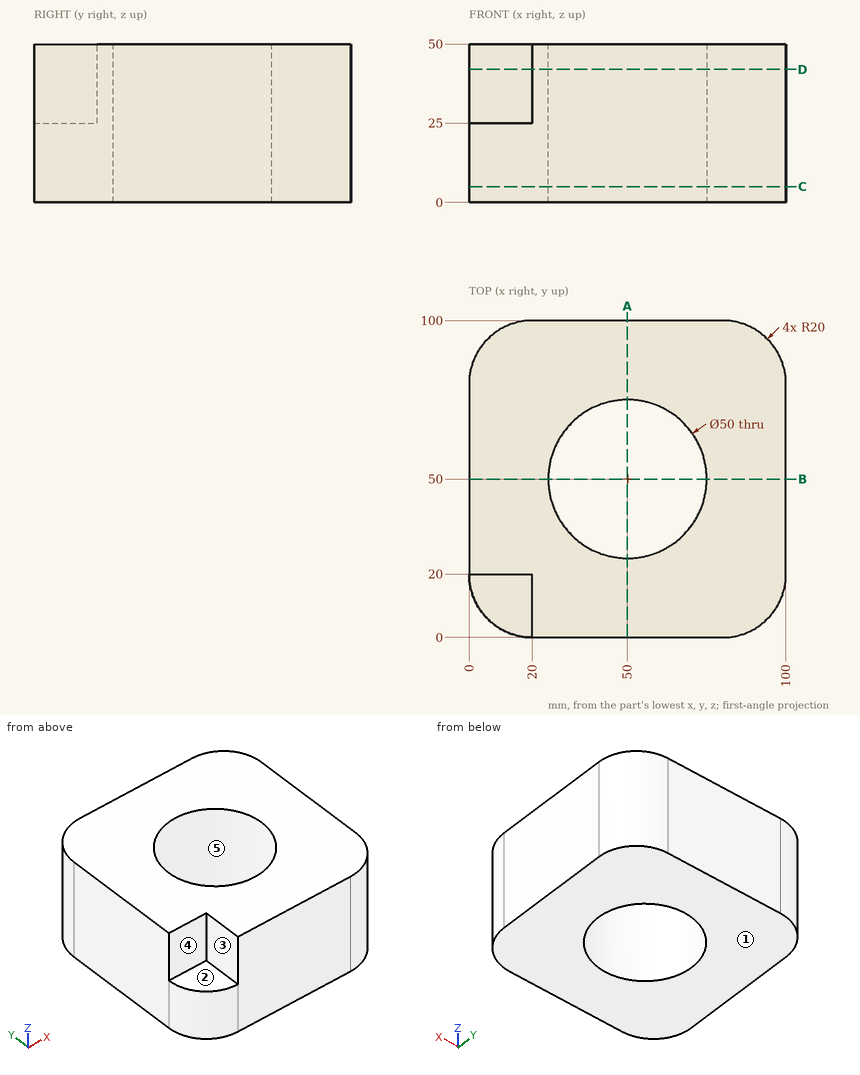
Verification items for this drawing (mm, ordinates from the low corner). A direction names the side the tool comes from. Give positions to 0.01 mm unless a question says otherwise; leave off trailing zeros. Loops run counter-clockwise (first coordinate to the right, second up) from the corner with the lowest first, then second, coordinate; pieces in that order, holes last. Notation, with made-up numbers: M 16.25,86 L 56.25,86 A16 cw 56.25,102 Z; hole C 84.25,-35.5 d3. An arc over 180 degrees is marked long. Answer as a JSON object with one key per item and string values. Group by question number.
Q1. Go/stop test with flat-tipped pins: P1, Ø6, axis at x = 7.5, y = 6.5, coming from the +Z side; P2, Ø12, axis at y = 11, z = 36, coming from the +X side; P3, Ø6, axis at x = 11.5, z = 36, coming from the -Y side. Record where each tip stops, or that it passes through.
Q2. Release check for a two-part mould opening along X. For the marked faces 3, 4 and 5 record: released by +X, released by -X, zero draft, split by the parting line, or undercut.
Q3. Access from +Z, -Z, +X, -X, +Y, -Y to the whole of each face (thin tool, end or side, straight path). Record for the marked faces 1 and 2.
Q4. Cross-section at A-A on x = 50. Record the cut outline in (y, z).
Q5. Material ranges on line 1 along Y through (x, z) = (50, 35.5); line 2 along X through (y, z) = (40.5, 35.5); line 3 along X through (y, z) = (65, 19), recorded low to high. Write a range as [from, to].
Q6. Cross-section at C-C on z = 5. Record the cut outline in (x, y), then the cut area to 3 significant figures.
Q7. Cross-section at D-D on z = 42. Record the cut outline in (x, y), then the cut area to 3 significant figures.
Evaluation:
{
 "1": {"P1": "stops at z = 25", "P2": "stops at x = 99.77", "P3": "stops at y = 20"},
 "2": {"face 3": "released by -X", "face 4": "zero draft", "face 5": "undercut"},
 "3": {"face 1": "-Z, +X, -X, +Y, -Y", "face 2": "+Z, -X, -Y"},
 "4": {"outline": "M 0,0 L 25,0 L 25,50 L 0,50 Z; M 75,0 L 100,0 L 100,50 L 75,50 Z"},
 "5": {"line 1": "y = [0, 25], [75, 100]", "line 2": "x = [0, 26.88], [73.12, 100]", "line 3": "x = [0, 30], [70, 100]"},
 "6": {"outline": "M 0,20 A20 ccw 20,0 L 80,0 A20 ccw 100,20 L 100,80 A20 ccw 80,100 L 20,100 A20 ccw 0,80 Z; hole C 50,50 d50", "area": "7,690 mm2"},
 "7": {"outline": "M 0,20 L 20,20 L 20,0 L 80,0 A20 ccw 100,20 L 100,80 A20 ccw 80,100 L 20,100 A20 ccw 0,80 Z; hole C 50,50 d50", "area": "7,380 mm2"}
}
